The listing builds one solid part. Answer for the finished solid, in the listing's coordinates (mm). Face numbers are marked on the shaded views. Coordinates: 2 decimals unless noted, no trailing zeros. Order: outer loops, then holes, each group sorted by start corner. A loop starts at its lowest first (then second) coordinate and runs counter-clockwise, first axis right, second up. Notation, with made-up numbers: (16, 69) - (64, 69) arc R15 cw to (64, 79) - close; hole circle Ø10 at (67.5, 52). An arc over 180 degrees is marked (long way). Use one line per item in the form item = value. Start each with the question number.
Item 1: Section A-A, the plane z = 0 is taken. Write down the section's boundary in (x, y), and give its area (3 significant figures).
Item 2: Each of these flat-tipped pins is pushed along its axis until it touches: pin 1 Ø2 at (x, z) = (8, 182.5) entering from +Y; pin 2 Ø10 at (x, y) = (27, 182.5) entering from +Z; pin 3 Ø1 at (x, y) = (13.5, 43) entering from +Z. Where does it stop, or does it pass through?
Item 3: The mould has two halves that part along Z. Classify the marked faces 1, 2 and 3: released by +Z, released by -Z, zero draft, split by the parting line, or undercut.
Item 4: Section C-C, the plane y = 0 is taken. Write down the section's boundary in (x, z).
Item 5: Consider line 1 along Z through (x, y) = (8, 46); line 2 along Y through (x, z) = (6, 59); line 3 along Y through (x, z) = (23.5, 101). Determine where each line is inside the solid, lowest interval first. Write a range as [from, to].
Item 6: Section D-D, the plane z = 130.5 is taken. Write down the section's boundary in (x, y), and give its area (3 significant figures).
Item 7: Section B-B, the plane x = 13 is taken. Write down the section's boundary in (y, z).
from build123d import *

# Parameters (mm, degrees)
SKETCH1_R           = 5
BOSS_EXTRUDE1_DEPTH = 30
SKETCH2_R           = 12.5
CUT_EXTRUDE1_DEPTH  = 20


with BuildPart() as part:
    # Sketch1 → Boss-Extrude1 (new body)
    with BuildSketch(Plane(origin=(0, 0, 0), x_dir=(0, 0, -1), z_dir=(1, 0, 0))):
        with BuildLine():
            Line((16.682027044, 11.032224332), (-107.430496688, 198.705028576))
            ThreePointArc((-107.430496688, 198.705028576), (-135.976276464, 217.975627767), (-169.787562283, 211.417084679))
            Line((-169.787562283, 211.417084679), (-232.345163698, 170.046243435))
            Line((-232.345163698, 170.046243435), (-210.280715034, 136.682189347))
            Line((-210.280715034, 136.682189347), (-181.087167707, 155.988581927))
            ThreePointArc((-181.087167707, 155.988581927), (-147.275881888, 162.547125016), (-118.730102112, 143.276525825))
            Line((-118.730102112, 143.276525825), (-16.682027044, -11.032224332))
            ThreePointArc((-16.682027044, -11.032224332), (11.032224332, -16.682027044), (16.682027044, 11.032224332))
        make_face()
        Circle(SKETCH1_R, mode=Mode.SUBTRACT)
    extrude(amount=BOSS_EXTRUDE1_DEPTH)

    # Sketch2 → Cut-Extrude1 (cut)
    with BuildSketch(Plane(origin=(0, -55.161121659, 83.41013522), x_dir=(1, 0, 0), z_dir=(0, -0.551611217, 0.834101352))):
        with Locations((15, 250)):
            Circle(SKETCH2_R)
    extrude(amount=-CUT_EXTRUDE1_DEPTH, mode=Mode.SUBTRACT)


solid = part.part
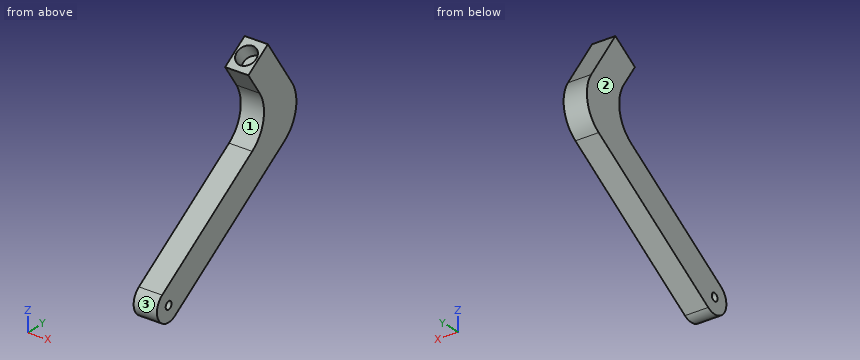
Response:
q1.outline = (0, -20) - (30, -20) - (30, -5) - (0, -5) - close; (0, 5) - (30, 5) - (30, 36.26) - (0, 36.26) - close
q1.area = 1,390 mm2
q2.pin_1 = 203.67
q2.pin_2 = 221.07
q2.pin_3 = 52.75
q3.face_1 = undercut
q3.face_2 = zero draft
q3.face_3 = split by the parting line
q4.outline = (0, -20) - (30, -20) - (30, -5) - (0, -5) - close; (0, 5) - (30, 5) - (30, 23.98) - (0, 23.98) - close
q5.line_1 = [6.44, 54.4]
q5.line_2 = [52.96, 125.47]
q5.line_3 = [116.47, 188.98]
q6.outline = (0, 155.35) - (30, 155.35) - (30, 216.49) - (0, 216.49) - close
q6.area = 1,830 mm2
q7.outline = (-11.03, 16.68) arc R20 ccw to (11.03, -16.68) - (198.71, 107.43) arc R45 ccw to (211.42, 169.79) - (170.05, 232.35) - (163.66, 228.12) - (174.69, 211.44) - (154.1, 197.82) - (143.07, 214.51) - (136.68, 210.28) - (155.99, 181.09) arc R45 cw to (143.28, 118.73) - close; hole circle Ø10 at (0, 0)
